```python
from build123d import *

# Parameters (mm, degrees)
F2_SIZE = 0.99999
F3_R    = 3
F4_R    = 1
F5_R    = 0.99999


# Not quite as in the source:
# - a fillet or chamfer is up to 0.001 mm smaller than in the source, because OpenCascade refuses the exact size


with BuildPart() as f1:
    # F0 (on Front) → F1 (revolve)
    with BuildSketch(Plane.XZ):
        Polygon((0, 2), (0, 0), (10.6, 0), (10.6, -1), (30, -1), (35, 60), (37.5, 73), (37.5, 96), (35.5, 96), (35.5, 73.1905618359), (33.0155331198, 60.2713340591), (28.1572270494, 1), (12.6, 1), (12.6, 2), align=None)
    revolve(axis=Axis((0, 0, 49), (0, 0, 1)))

    # F2 (size 1 in the source; OpenCascade refuses exactly that, so slightly less here)
    f2_edges = [f1.edges().sort_by_distance(p)[0] for p in [
        (-10.6, 0, -1),
    ]]
    chamfer(f2_edges, length=F2_SIZE)

    # F3
    f3_edges = [f1.edges().sort_by_distance(p)[0] for p in [
        (-30, 0, -1),
    ]]
    fillet(f3_edges, radius=F3_R)

    # F4
    f4_edges = [f1.edges().sort_by_distance(p)[0] for p in [
        (-28.157227, 0, 1),
    ]]
    fillet(f4_edges, radius=F4_R)

    # F5 (radius 1 in the source; OpenCascade refuses exactly that, so slightly less here)
    f5_edges = [f1.edges().sort_by_distance(p)[0] for p in [
        (-12.6, 0, 1),
    ]]
    fillet(f5_edges, radius=F5_R)


solid = f1.part
```
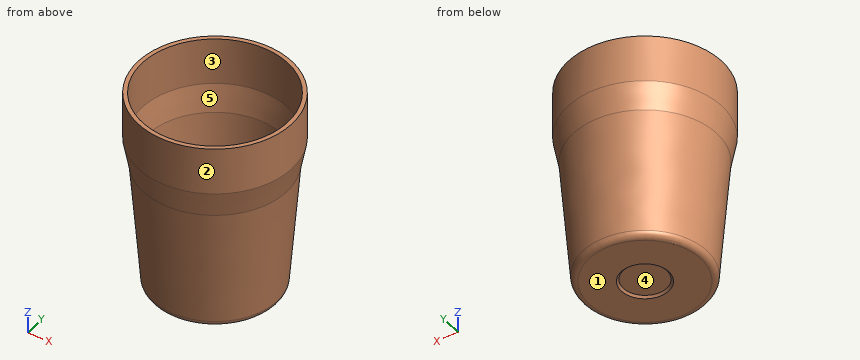
Read the model definition and answer for the solid it produces. Units are mm, in the model's axes. Face numbers are marked on the shaded views. A direction names the side the tool comes from. Give positions to 0.01 mm unless a question says otherwise; leave off trailing zeros. Loops run counter-clockwise (first coordinate to the right, second up) from the corner with the lowest first, then second, coordinate; pieces in that order, holes last.
Item 1: The part is cut by section C-C (z = 83.5). Write down the section's boundary in (x, y).
Item 2: The part is cut by section D-D (z = 34.5). Write down the section's boundary in (x, y), and give its area (3 significant figures).
Item 3: For the marked faces 4 and 5, determine the directions among +Z, -Z, +X, -X, +Y, -Y from which every point of the face is accessible in a straight line to the end or side of a thin tool.
Item 4: Each of these flat-tipped pins is pushed along its axis until it touches: pin 1 Ø1 at (x, y) = (6.5, 1) entering from +Z; pin 2 Ø4 at (x, z) = (-9.5, 54) entering from +Y; pin 3 Ø19 at (x, y) = (0, 0) entering from -Z. Where does it stop, or does it pass through?
Item 5: Find the intervals of material crossed by line 1 along Y through (x, z) = (0, 88.5); line 2 along Z through (x, y) = (-19, -1); line 3 along Y through (x, z) = (8.5, 39), in increasing order.
Item 6: The mould has two halves that part along Y. Classify the marked faces 1, 2 and 3: released by +Y, released by -Y, zero draft, split by the parting line, or undercut.
Taken from the geometry:
1. outline: circle Ø75 at (0, 0); hole circle Ø71 at (0, 0)
2. outline: circle Ø65.82 at (0, 0); hole circle Ø61.81 at (0, 0)
2. area: 402 mm2
3. face 4: -Z
3. face 5: +Z
4. pin 1: stops at z = 2
4. pin 2: stops at y = 33.71
4. pin 3: stops at z = 0
5. line 1: y = -37.5 to -35.5, 35.5 to 37.5
5. line 2: z = -1 to 1
5. line 3: y = -32.17 to -30.09, 30.09 to 32.17
6. face 1: zero draft
6. face 2: split by the parting line
6. face 3: undercut
